Design review of the part built by this model. Coordinates are the model's own, in mm. A direction names the side the tool comes from. Coordinates: 2 decimals unless noted, no trailing zeros. Order: outer loops, then holes, each group sorted by start corner. A loop starts at its lowest first (then second) coordinate and runs counter-clockwise, first axis right, second up.
Autodesk Inventor part; units mm, degrees
ref_plane "YZ Plane" through (0, 0, 0) normal (1, 0, 0) x (0, 1, 0)
ref_plane "XZ Plane" through (0, 0, 0) normal (0, 1, 0) x (-1, 0, 0)
ref_plane "XY Plane" through (0, 0, 0) normal (0, 0, 1) x (1, 0, 0)
sketch "Sketch1" plane through (0, 0, 0) normal (0, 1, 0) x (-1, 0, 0)
  line L0 (-27.5, -7.5) -> (-52.5, -7.5) construction
  line L1 (-27.5, -5) -> (-52.5, -5)
  line L2 (-52.5, -10) -> (-27.5, -10)
  arc A0 (-27.5, -10) -> (-27.5, -5) centre (-27.5, -7.5) ccw
  arc A1 (-52.5, -5) -> (-52.5, -10) centre (-52.5, -7.5) ccw
  line L3 (-4, -12) -> (-76, -12)
  line L4 (-80, -8) -> (-80, 0)
  line L5 (-80, 0) -> (0, 0)
  line L6 (0, 0) -> (0, -8)
  arc A2 (-4, -12) -> (0, -8) centre (-4, -8) ccw
  arc A3 (-80, -8) -> (-76, -12) centre (-76, -8) ccw
  point P0 (-40, -7.5)
  point P1 (-80, -12)
  point P2 (-40, -12)
  dimension "d0" = 25
  dimension "d1" = 5
  dimension "d2" = 80
  dimension "d3" = 12
  dimension "d5" = 4
  dimension "d6" = 2
extrude "Extrusion1" add sketch "Sketch1" along normal blind 2
sketch "Sketch2" plane through (0, 0, 0) normal (0, 0, 1) x (1, 0, 0)
  circle A0 centre (6, 7) radius 1.5
  circle A1 centre (74, 7) radius 1.5
  line L0 (0, 0) -> (0, 2)
  line L1 (80, 0) -> (80, 2)
  line L2 (0, 2) -> (80, 2)
  line L3 (4, 2) -> (0, 2)
  line L4 (76, 2) -> (4, 2)
  line L5 (9.2479, 2) -> (12, 2)
  arc A2 (8.6585, 5.6098) -> (3.3415, 8.3902) centre (6, 7) ccw
  line L6 (0, 2) -> (3.3415, 8.3902)
  line L7 (7.9187, 4.1951) -> (8.6585, 5.6098)
  arc A3 (7.9187, 4.1951) -> (9.2479, 2) centre (9.2479, 3.5) ccw
  arc A4 (76.6585, 8.3902) -> (71.3415, 5.6098) centre (74, 7) ccw
  line L8 (80, 2) -> (76.6585, 8.3902)
  line L9 (71.3415, 5.6098) -> (72.0813, 4.1951)
  line L10 (70.7521, 2) -> (70.1315, 2)
  arc A5 (70.7521, 2) -> (72.0813, 4.1951) centre (70.7521, 3.5) ccw
  point P0 (6.7708, 2)
  point P1 (73.2292, 2)
  point P2 (9.2479, 2)
  dimension "d9" = 3
  dimension "d10" = 3
  dimension "d11" = 6
  dimension "d12" = 6
  dimension "d13" = 5
  dimension "d16" = 6
  dimension "d17" = 1.5
  dimension "d18" = 6
  dimension "d19" = 1.5
extrude "Extrusion2" add sketch "Sketch2" against normal blind 2
fillet "Fillet1" radius 2 2 edges at (0, 1, 0) (80, 1, 0)
equation "\"d10\" = d9"
equation "\"d12\" = d11"
equation "\"d18\" = d16"
equation "\"d19\" = d17"
properties part number "PCB Mount Support"
1. For faces 4 (the flat face through (75, 5, -2)), 5 (the cylindrical face through (79.13, 1.66, -0.35)), 6 (the cylindrical face through (25, 1, -7.4)), 7 (the flat face through (39, 1, -12)), 8 (the flat face through (8.28, 4.89, -0.99)), list the 3-axis set-ups (+Z, -Z, +X, -X, +Y, -Y) from which the entire face can be reached by the end or side of a thin tool; tool diameter is ignored.
2. To check wall thickness, follow line 1 (Y direction, x = 6, z = -1.25); line 2 (Y direction, x = 14, z = -3.25); line 3 (X direction, y = 0.75, z = -9). State the ranges of each line that lie inside material, in increasing order.
3. Add section D-D (x = 6). Give the boundary of the cut face in (y, z).
4. Add section C-C (z = -7). Give the boundary of the cut face in (x, y), and give its area (3 significant figures).
5. Insertion check: pin 1 (4 mm diameter, centred on x = 26, y = 4.5, fed in from +Z); pin 2 (4 mm diameter, centred on x = 61, z = -10.5, fed in from +Y); pin 3 (3.5 mm diameter, centred on x = 74, y = 7, fed in from -Z). Each pin has a flat end and moves straight along its axis. Give the tip position at first contact, or say it passes through.
6. Add section B-B (y = 7). Give the boundary of the cut face in (x, z), and give its area (3 significant figures).
7. Mouldability with a two-part tool opening along Y and no side actions: class faces 1 (the flat face through (77.98, 5.86, -0.99)), 2 (the cylindrical face through (72.02, 2.7, -0.99)), 3 (the cylindrical face through (78.797, 0.986, -10.859)) as pulls with the +Y half, pulls with the -Y half, needs draft (parallel to the pull), parting line crosses it, or undercut.
8. Add section A-A (x = 49.5). Give the boundary of the cut face in (y, z).
Solution:
1. face 4: -Z, +X, -X, +Y
1. face 5: +Z, +X, +Y, -Y
1. face 6: +Y, -Y
1. face 7: -Z, +X, -X, +Y, -Y
1. face 8: +Z, -Z
2. line 1: y = 0 to 5.5, 8.5 to 10
2. line 2: y = 0 to 2
2. line 3: x = 0.13 to 25.5, 54.5 to 79.87
3. outline: (0, -12) - (2, -12) - (2, -2) - (5.5, -2) - (5.5, 0) - (0, 0) - close; (8.5, -2) - (10, -2) - (10, 0) - (8.5, 0) - close
4. outline: (0, 0) - (25.05, 0) - (25.05, 2) - (0, 2) - close; (54.95, 0) - (80, 0) - (80, 2) - (54.95, 2) - close
4. area: 100 mm2
5. pin 1: passes through
5. pin 2: stops at y = 2
5. pin 3: stops at z = -2
6. outline: (2.61, -2) - (4.5, -2) - (4.5, 0) - (2.61, 0) - close; (7.5, -2) - (9, -2) - (9, 0) - (7.5, 0) - close; (71, -2) - (72.5, -2) - (72.5, 0) - (71, 0) - close; (75.5, -2) - (77.39, -2) - (77.39, 0) - (75.5, 0) - close
6. area: 13.5 mm2
7. face 1: pulls with the +Y half
7. face 2: undercut
7. face 3: needs draft
8. outline: (0, -12) - (2, -12) - (2, -10) - (0, -10) - close; (0, -5) - (2, -5) - (2, 0) - (0, 0) - close
